Work out the finished part from the listing and answer in its coordinate system (mm). A direction names the side the tool comes from. Coordinates: 2 decimals unless noted, no trailing zeros. Order: outer loops, then holes, each group sorted by start corner. A loop starts at its lowest first (then second) coordinate and runs counter-clockwise, first axis right, second up. Notation, with made-up numbers: (-39, 0.25) - (-4, 0.25) arc R16 ccw to (-4, 9.25) - close; hole circle Ø2 at (75.25, -5.5). An arc over 180 degrees is marked (long way). Answer as a JSON object with one key per item and string values. Group by question number.
1) Each of these flat-tipped pins is pushed along its axis until it touches: P1, Ø1.5, axis at y = 6, z = 1.5, coming from the +X side; P2, Ø0.9, axis at y = 5, z = 0.5, coming from the -X side; P3, Ø6.5, axis at x = 1, z = 2, coming from the -Y side. Where does it stop, or does it pass through?
2) A tool of negligible diameter and unlimited length cuts with its end or side. For faces 1 (the face through (5, -1, 0)), 2 (the face through (-3, 2, 1)), 3 (the face through (-1.8, 5, 0)), from which of +Z, -Z, +X, -X, +Y, -Y can it reach the whole face along a straight path? Write none if from no direction.
3) Section A-A (x = 0) is taken. Give the vertices of the cut face in (y, z), plus the area to 3 significant figures.
4) Section C-C (y = 2) is taken. Give the vertices of the cut face in (x, z), plus the area to 3 significant figures.
5) Find the intervals of material crossed by line 1 along X through (y, z) = (0.75, 5); line 2 along X through (y, z) = (-0.75, 2); line 3 along Z through (x, y) = (0, 6.25), in increasing order.
6) Section B-B (y = -1) is taken. Give the vertices of the cut face in (x, z), plus the area to 3 significant figures.
7) The mould has two halves that part along Y. Classify faces 4 (the face through (-5.2, -3.3, -0.1)), 5 (the face through (3.4, 0, 0.1)), 6 (the face through (5.297, 5.859, -0.08)), 7 (the face through (-0.04, 5.48, -3.35)): released by +Y, released by -Y, zero draft, split by the parting line, or undercut.
8) Section D-D (y = 5.25) is taken. Give the vertices of the cut face in (x, z).
Autodesk Inventor part; units mm, degrees
ref_plane "YZ Plane" through (0, 0, 0) normal (1, 0, 0) x (0, 1, 0)
ref_plane "XZ Plane" through (0, 0, 0) normal (0, 1, 0) x (-1, 0, 0)
ref_plane "XY Plane" through (0, 0, 0) normal (0, 0, 1) x (1, 0, 0)
sketch "Sketch1" plane through (0, 0, 0) normal (0, 1, 0) x (-1, 0, 0)
  line L0 (6.5, 5.75) -> (-6.5, 5.75)
  line L1 (-6.5, 5.75) -> (-6.5, -5.75)
  line L2 (-6.5, -5.75) -> (6.5, -5.75)
  line L3 (6.5, -5.75) -> (6.5, 5.75)
  line L4 (6.5, 5.75) -> (-6.5, -5.75) construction
  line L5 (-6.5, 5.75) -> (6.5, -5.75) construction
  point P0 (0, 0)
  dimension "d0" = 13
  dimension "d1" = 11.5
extrude "Extrusion1" add sketch "Sketch1" along normal blind 7
sketch "Sketch2" plane through (0, 0, 0) normal (0, -1, 0) x (1, 0, 0)
  line L0 (3, 5.75) -> (-3, 5.75)
  line L1 (-3, 5.75) -> (-3, -4.75)
  line L2 (-3, -4.75) -> (3, -4.75)
  line L3 (3, -4.75) -> (3, 5.75)
  line L4 (3, 5.75) -> (-3, -4.75) construction
  line L5 (-3, 5.75) -> (3, -4.75) construction
  line L6 (-6.5, 5.75) -> (6.5, 5.75)
  point P0 (0, 0)
  point P1 (0, 0.5)
  dimension "d4" = 6
  dimension "d5" = 10.5
extrude "Extrusion2" cut sketch "Sketch2" against normal blind 4
sketch "Sketch4" plane through (0, 4, 0) normal (0, -1, 0) x (1, 0, 0)
  line L0 (0, 4.25) -> (0, -3.35) construction
  line L1 (-1.8, 2.45) -> (-1.8, -1.55)
  line L2 (1.8, -1.55) -> (1.8, 2.45)
  arc A0 (1.8, 2.45) -> (-1.8, 2.45) centre (0, 2.45) ccw
  arc A1 (-1.8, -1.55) -> (1.8, -1.55) centre (0, -1.55) ccw
  line L3 (-3, 5.75) -> (3, 5.75)
  point P0 (0, 0)
  point P1 (0, 0.45)
  dimension "d15" = 3.6
  dimension "d16" = 4
  dimension "d17" = 3.3
extrude "Extrusion4" cut sketch "Sketch4" against normal blind 3
sketch "Sketch5" plane through (0, 0, 0) normal (0, -1, 0) x (1, 0, 0)
  line L0 (6.5, 5.75) -> (6.5, -5.75)
  line L1 (3, 5.75) -> (6.5, 5.75)
  line L2 (6.5, -5.75) -> (5, -5.75)
  line L3 (5, -5.75) -> (5, 5.75)
  line L4 (5, 5.75) -> (6.5, 5.75)
  line L5 (6.5, 5.75) -> (6.5, -5.75)
  line L6 (-6.5, -5.75) -> (-6.5, 5.75)
  line L7 (-6.5, 5.75) -> (-3, 5.75)
  line L8 (-6.5, -5.75) -> (-5, -5.75)
  line L9 (-5, -5.75) -> (-5, 5.75)
  line L10 (-5, 5.75) -> (-6.5, 5.75)
  line L11 (-6.5, 5.75) -> (-6.5, -5.75)
  point P0 (0, 0)
  dimension "d24" = 1.5
  dimension "d25" = 1.5
extrude "Extrusion5" add sketch "Sketch5" along normal blind 2
sketch "Sketch6" plane through (0, -2, 0) normal (0, -1, 0) x (1, 0, 0)
  line L0 (6.5, 5.75) -> (6.5, -5.75)
  line L1 (6.5, -5.75) -> (4.5, -5.75)
  line L2 (4.5, -5.75) -> (4.5, 5.75)
  line L3 (4.5, 5.75) -> (6.5, 5.75)
  line L4 (6.5, 5.75) -> (6.5, -5.75)
  line L5 (-6.5, -5.75) -> (-6.5, 5.75)
  line L6 (-6.5, -5.75) -> (-4.5, -5.75)
  line L7 (-4.5, -5.75) -> (-4.5, 5.75)
  line L8 (-4.5, 5.75) -> (-6.5, 5.75)
  line L9 (-6.5, 5.75) -> (-6.5, -5.75)
  point P0 (0, 0)
  dimension "d28" = 2
  dimension "d29" = 2
extrude "Extrusion6" add sketch "Sketch6" along normal blind 2
chamfer "Chamfer2" distance 1.4 angle 45 2 edges at (4.5, -4, 0) (-4.5, -4, 0)
fillet "Fillet2" radius 1 2 edges at (4.5, -2.6, 0) (-4.5, -2.6, 0)
fillet "Fillet3" radius 0.5 4 edges at (6.5, -4, 0) (5.9, -4, 0) (-6.5, -4, 0) (-5.9, -4, 0)
fillet "Fillet4" radius 4 2 edges at (6.5, 7, 0) (-6.5, 7, 0)
properties part number "IR_Focus_Dark"
Report:
{
 "1": {"P1": "stops at x = 5.81", "P2": "stops at x = -6.19", "P3": "stops at y = 0"},
 "2": {"face 1": "+Z, -Z", "face 2": "+Z, -Y", "face 3": "+Y, -Y"},
 "3": {"outline": "(0, -5.75) - (7, -5.75) - (7, -3.35) - (4, -3.35) - (4, -4.75) - (0, -4.75) - close; (4, 4.25) - (7, 4.25) - (7, 5.75) - (4, 5.75) - close", "area": "15.7 mm²"},
 "4": {"outline": "(-6.5, -5.75) - (6.5, -5.75) - (6.5, 5.75) - (3, 5.75) - (3, -4.75) - (-3, -4.75) - (-3, 5.75) - (-6.5, 5.75) - close", "area": "86.5 mm²"},
 "5": {"line 1": "x = -6.5 to -3, 3 to 6.5", "line 2": "x = -6.5 to -5, 5 to 6.5", "line 3": "z = -5.75 to -3.35, 4.25 to 5.75"},
 "6": {"outline": "(-6.5, -5.75) - (-5, -5.75) - (-5, 5.75) - (-6.5, 5.75) - close; (5, -5.75) - (6.5, -5.75) - (6.5, 5.75) - (5, 5.75) - close", "area": "34.5 mm²"},
 "7": {"face 4": "released by -Y", "face 5": "undercut", "face 6": "released by +Y", "face 7": "zero draft"},
 "8": {"outline": "(-5.81, -5.75) - (5.81, -5.75) - (5.81, 5.75) - (-5.81, 5.75) - close; hole (-1.8, -1.55) arc R1.8 ccw to (1.8, -1.55) - (1.8, 2.45) arc R1.8 ccw to (-1.8, 2.45) - close"}
}
